Read the model definition and answer for the solid it produces. Units are mm, in the model's axes. Round coordinates to 2 decimals unless told otherwise and drop trailing zeros. Write each loop counter-clockwise with the first axis right and the second up, starting at its lowest first coordinate (ties: lowest second). Pieces come first, ordered by that corner, then holes. Notation, with made-up numbers: (-40, 21.25) -> (-1, 21.25) arc R33 ccw to (-1, 52.25) -> close; hole circle Ø1 at (78, -8). An arc over 180 degrees is marked (long way). Return JSON: item names as keys, results as strings.
Autodesk Inventor part; units mm, degrees
ref_plane "YZ Plane" through (0, 0, 0) normal (1, 0, 0) x (0, 1, 0)
ref_plane "XZ Plane" through (0, 0, 0) normal (0, 1, 0) x (-1, 0, 0)
ref_plane "XY Plane" through (0, 0, 0) normal (0, 0, 1) x (1, 0, 0)
sketch "Sketch1" plane through (0, 0, 0) normal (0, 0, 1) x (1, 0, 0)
  circle A0 centre (0, 0) radius 50
  dimension "d0" = 100
extrude "Extrusion1" add sketch "Sketch1" along normal blind 5
sketch "Sketch2" plane through (0, 0, 5) normal (0, 0, 1) x (1, 0, 0)
  circle A0 centre (0, 0) radius 24
  dimension "d3" = 48
extrude "Extrusion2" cut sketch "Sketch2" against normal blind 5
sketch "Sketch3" plane through (0, 0, 5) normal (0, 0, 1) x (1, 0, 0)
  circle A0 centre (0, 42.5) radius 3.5
  circle A1 centre (0, 0) radius 50
  circle A2 centre (-36.8061, -21.25) radius 3.5
  circle A3 centre (36.8061, -21.25) radius 3.5
  dimension "d6" = 7
  dimension "d8" = 4
  dimension "d11" = 360
extrude "Extrusion3" cut sketch "Sketch3" against normal blind 5 contours A0 | A2 | A3
properties part number "blacha pod odciągi"
Item 1: Section C-C (z = 2.15) is taken. Give the vertices of the cut face in (x, y), then the cut area to 3 significant figures.
Worked answers:
{"outline": "circle Ø100 at (0, 0); hole circle Ø7 at (-36.81, -21.25); hole circle Ø48 at (0, 0); hole circle Ø7 at (0, 42.5); hole circle Ø7 at (36.81, -21.25)", "area": "5,930 mm2"}
Item 2: Section D-D (x = 37) is taken. Give the vertices of the cut face in (y, z).
Worked answers:
{"outline": "(-33.63, 0) -> (-24.74, 0) -> (-24.74, 5) -> (-33.63, 5) -> close; (-17.76, 0) -> (33.63, 0) -> (33.63, 5) -> (-17.76, 5) -> close"}
Item 3: A flat-ended cylindrical pin translates along its axis: pin 1 (8 mm diameter, centred on x = 36.81, y = -21.25, fed in from -Z). Find the tip coordinate at first contact, or state that the pin passes through.
Worked answers:
{"pin 1": "stops at z = 0"}
Item 4: Section A-A (y = 0) is taken. Give the vertices of the cut face in (x, z), then the cut area to 3 significant figures.
Worked answers:
{"outline": "(-50, 0) -> (-24, 0) -> (-24, 5) -> (-50, 5) -> close; (24, 0) -> (50, 0) -> (50, 5) -> (24, 5) -> close", "area": "260 mm2"}
Item 5: Straight lines are drawn through the part: L1, parallel to Y at x = 0, z = 3.8; L2, parallel to Y at x = 1, z = 3.3; L3, parallel to Y at x = -13, z = 2.55. For each, find the intervals that lie inside material, in ascending order. Write a range as [from, to].
Worked answers:
{"L1": "y = [-50, -24], [24, 39], [46, 50]", "L2": "y = [-49.99, -23.98], [23.98, 39.15], [45.85, 49.99]", "L3": "y = [-48.28, -20.17], [20.17, 48.28]"}
Item 6: Section B-B (x = 0) is taken. Give the vertices of the cut face in (y, z), then the cut area to 3 significant figures.
Worked answers:
{"outline": "(-50, 0) -> (-24, 0) -> (-24, 5) -> (-50, 5) -> close; (24, 0) -> (39, 0) -> (39, 5) -> (24, 5) -> close; (46, 0) -> (50, 0) -> (50, 5) -> (46, 5) -> close", "area": "225 mm2"}
Item 7: For a pull along Y with two mould halves and no side action, classify faces 1 (the cylindrical face through (-37.26, -17.78, 2.54)), 2 (the cylindrical face through (47.69, -15.02, 2.46)), 3 (the flat face through (22, 12, 0)) as released by +Y, released by -Y, zero draft, split by the parting line, or undercut.
Worked answers:
{"face 1": "undercut", "face 2": "split by the parting line", "face 3": "zero draft"}
